Design review of the part built by this model. Coordinates are the model's own, in mm. Face numbers are marked on the shaded views. Round coordinates to 2 decimals unless told otherwise and drop trailing zeros. Loops run counter-clockwise (first coordinate to the right, second up) from the corner with the lowest first, then second, coordinate; pieces in that order, holes last. Notation, with made-up numbers: M -39,1 L -26,1 A13 ccw -26,14 Z; hole C 80,13.25 d4. An arc over 180 degrees is marked long. Use a Markdown table: item, result.
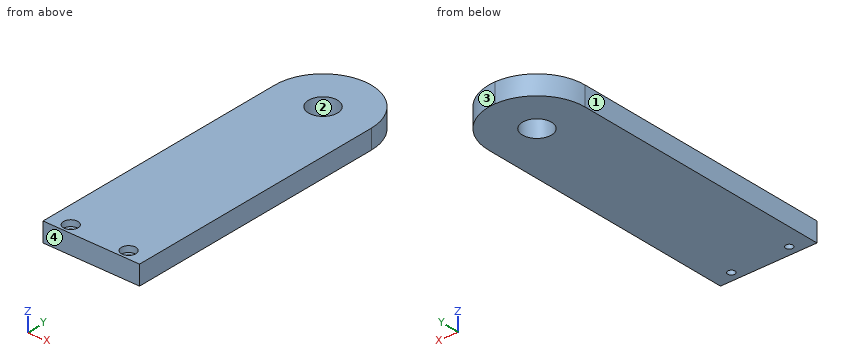
Autodesk Inventor part; units mm, degrees
ref_plane "YZ Plane" through (0, 0, 0) normal (1, 0, 0) x (0, 1, 0)
ref_plane "XZ Plane" through (0, 0, 0) normal (0, 1, 0) x (-1, 0, 0)
ref_plane "XY Plane" through (0, 0, 0) normal (0, 0, 1) x (1, 0, 0)
sketch "Sketch1" plane through (0, 0, 0) normal (0, 0, 1) x (1, 0, 0)
  circle A0 centre (0, 0) radius 6
  line L0 (20, 20) -> (20, -20)
  line L1 (20, -20) -> (-20, -20)
  line L2 (-20, -20) -> (-20, 20)
  line L3 (-20, 20) -> (20, 20)
  line L4 (-20, -20) -> (20, -20)
  line L5 (20, -20) -> (20, -110)
  line L6 (20, -110) -> (-20, -110)
  line L7 (-20, -110) -> (-20, -20)
  dimension "d0" = 12
  dimension "d1" = 40
  dimension "d5" = 110
extrude "Extrusion1" add sketch "Sketch1" along normal blind 8
fillet "Fillet1" radius 20 2 edges at (20, 20, 4) (-20, 20, 4)
sketch "Sketch2" plane through (0, 0, 8) normal (0, 0, 1) x (1, 0, 0)
  line L0 (20, -110) -> (-20, -110) construction
  line L1 (-20, -110) -> (-20, 0) construction
  line L2 (20, 0) -> (20, -110) construction
  line L3 (-20, -110) -> (20, -110) construction
  line L4 (20, -110) -> (20, -102) construction
  line L5 (20, -102) -> (-20, -102) construction
  line L6 (-20, -102) -> (-20, -110) construction
  line L7 (0, -102) -> (0, -110) construction
  line L8 (0, -106) -> (-12, -106) construction
  circle A0 centre (-12, -106) radius 1.5
  point P0 (0, 0)
  dimension "d7" = 8
  dimension "d8" = 3
  dimension "d14" = 12
extrude "Extrusion2" cut sketch "Sketch2" against normal through all
sketch "Sketch3" plane through (0, 0, 8) normal (0, 0, 1) x (1, 0, 0)
  circle A0 centre (-12, -106) radius 1.5
  circle A1 centre (-12, -106) radius 3
  point P0 (0, 0)
  dimension "d11" = 6
extrude "Extrusion3" cut sketch "Sketch3" against normal blind 2.5
mirror "Mirror1" about plane through (0, 0, 0) normal (1, 0, 0) of "Extrusion2", "Extrusion3"
properties part number "Bearing10"
1. Wall thickness on line 1 along Y through (x, z) = (0, 5); line 2 along X through (y, z) = (-106, 3.5); line 3 along X through (y, z) = (-104, 7): over which ranges is each line inside the solid? List them lowest first. Write a range as from..to.
Check values:
| item | result |
|---|---|
| line 1 | y = -110..-6, 6..20 |
| line 2 | x = -20..-13.5, -10.5..10.5, 13.5..20 |
| line 3 | x = -20..-14.24, -9.76..9.76, 14.24..20 |
2. Take a section at B-B on x = -12. Give the boundary of the cut face in (y, z), and give its area (4 significant figures).
Check values:
| item | result |
|---|---|
| outline | M -110,0 L -107.5,0 L -107.5,5.5 L -109,5.5 L -109,8 L -110,8 Z; M -104.5,0 L 16,0 L 16,8 L -103,8 L -103,5.5 L -104.5,5.5 Z |
| area | 976.5 mm² |
3. Take a section at A-A on z = 2.25. Count the separate pieces of the cut face and the enclosed holes in it, and give its area (3 significant figures).
Check values:
| item | result |
|---|---|
| separate pieces | 1 |
| enclosed holes | 3 |
| area | 4,900 mm² |
4. Insertion check: pin 1 (5 mm diameter, centred on x = -12, y = -106, fed in from +Z). The pin has a flat end and moves straight along its axis. Give the tip position at first contact, or say it passes through.
Check values:
| item | result |
|---|---|
| pin 1 | stops at z = 5.5 |
5. The part is to be moulded in two halves that separate along X. For the marked faces 1, 2, 3 and 4, say which applies: pulls with the +X half, pulls with the -X half, needs draft (parallel to the pull), parting line crosses it, or undercut.
Check values:
| item | result |
|---|---|
| face 1 | pulls with the -X half |
| face 2 | undercut |
| face 3 | pulls with the +X half |
| face 4 | needs draft |
6. Take a section at C-C on x = 17. Give the boundary of the cut face in (y, z).
Check values:
| item | result |
|---|---|
| outline | M -110,0 L 10.54,0 L 10.54,8 L -110,8 Z |
